```python
from build123d import *

# Parameters (mm, degrees)
SKETCH1_W           = 18.4
SKETCH1_H           = 46.99
SKETCH1_W_2         = 2.05
SKETCH1_H_2         = 2.05
SKETCH1_W_3         = 3.175
BOSS_EXTRUDE1_DEPTH = 3.175
SKETCH2_W           = 3.175
SKETCH2_H           = 46.99
CUT_EXTRUDE1_DEPTH  = 4.175


with BuildPart() as part:
    # Sketch1 → Boss-Extrude1 (new body)
    with BuildSketch(Plane(origin=(0, 0, 0), x_dir=(1, 0, 0), z_dir=(0, 1, 0))):
        Rectangle(SKETCH1_W, SKETCH1_H)
        with Locations((0, -18.93924342)):
            Rectangle(SKETCH1_W_2, SKETCH1_H_2, mode=Mode.SUBTRACT)
        with Locations((-10.7875, 0)):
            Rectangle(SKETCH1_W_3, SKETCH1_H)
    extrude(amount=BOSS_EXTRUDE1_DEPTH)

    # Sketch2 → Cut-Extrude1 (cut, through all)
    with BuildSketch(Plane(origin=(0, 3.175, 0), x_dir=(1, 0, 0), z_dir=(0, 1, 0))):
        with Locations((-10.7875, 0)):
            Rectangle(SKETCH2_W, SKETCH2_H)
    extrude(amount=-CUT_EXTRUDE1_DEPTH, mode=Mode.SUBTRACT)


solid = part.part
```
The listing builds one solid part. Answer for the finished solid, in the listing's coordinates (mm). A direction names the side the tool comes from. Round coordinates to 2 decimals unless told otherwise and drop trailing zeros. Loops run counter-clockwise (first coordinate to the right, second up) from the corner with the lowest first, then second, coordinate; pieces in that order, holes last. Notation, with made-up numbers: (-22, 12) -> (12, 12) arc R30 cw to (12, 39) -> close; hole circle Ø5 at (-1, 57.25). An arc over 180 degrees is marked (long way). Use one line per item in the form item = value.
1. The part is cut by section A-A on z = 19. Determine the outline of the cut face in (x, y) (3 decimals), and give its area (3 significant figures).
Answer key:
outline = (-9.2, 0) -> (-1.025, 0) -> (-1.025, 3.175) -> (-9.2, 3.175) -> close; (1.025, 0) -> (9.2, 0) -> (9.2, 3.175) -> (1.025, 3.175) -> close
area = 51.9 mm²
2. A tool of negligible diameter and unlimited length cuts with its end or side. For faces 4 (the flat face through (0, 2, 17.914)), 5 (the flat face through (9.2, 2, 0)), from which of +Z, -Z, +X, -X, +Y, -Y can it reach the whole face along a straight path? Write none if from no direction.
Answer key:
face_4 = +Y, -Y
face_5 = +Z, -Z, +X, +Y, -Y
3. Find the intervals of material crossed by probe 1 along Z at (x, y) = (-0.25, 0.35) (3 decimals), in increasing order. Write a range as [from, to].
Answer key:
probe_1 = [-23.495, 17.914], [19.964, 23.495]
4. For a pull along Z with two mould halves and no side action, classify faces 1 (the flat face through (-1.025, 2, 19)), 2 (the flat face through (0, 2, -23.495)), 3 (the flat face through (0, 2, 23.495)) as released by +Z, released by -Z, zero draft, split by the parting line, or undercut.
Answer key:
face_1 = undercut
face_2 = released by -Z
face_3 = released by +Z
5. The part is cut by section B-B on x = 0.5. Determine the outline of the cut face in (y, z) (3 decimals).
Answer key:
outline = (0, -23.495) -> (3.175, -23.495) -> (3.175, 17.914) -> (0, 17.914) -> close; (0, 19.964) -> (3.175, 19.964) -> (3.175, 23.495) -> (0, 23.495) -> close
